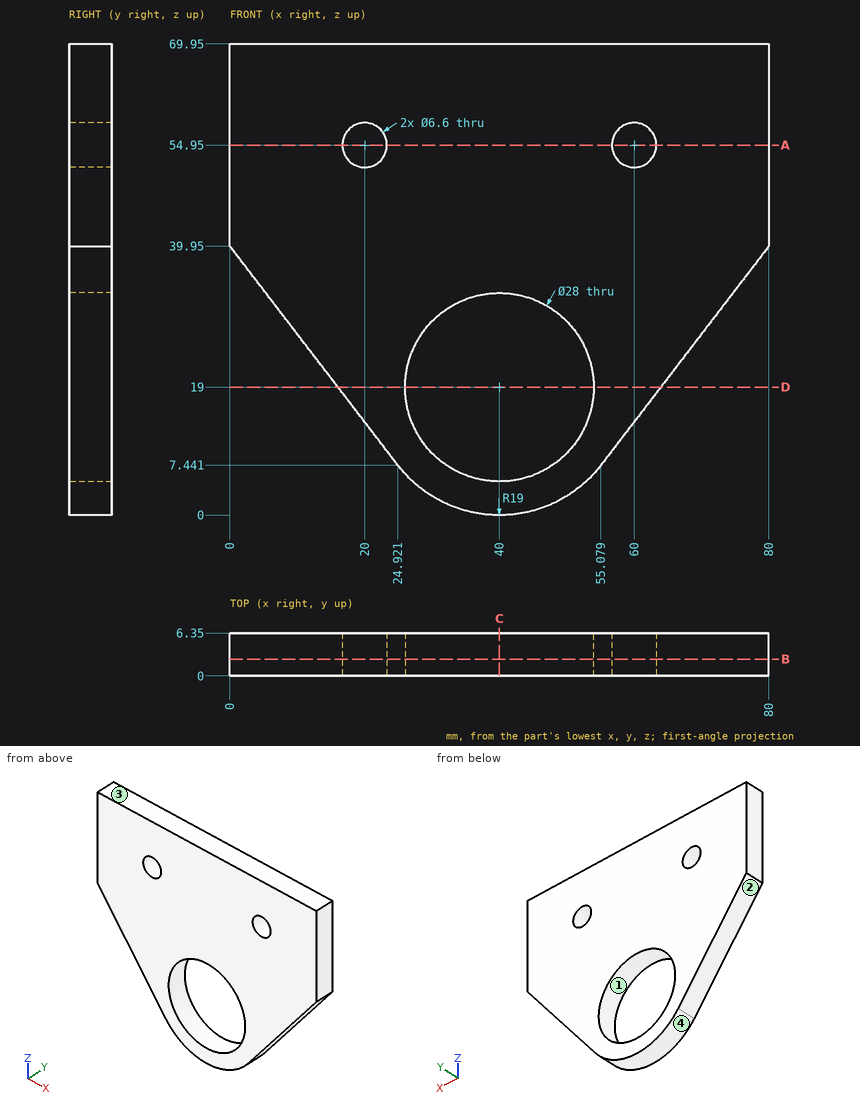
Can you work these out from the drawing? Everything is in mm from the part's minimum corner. Round coordinates to 2 decimals unless told otherwise and drop trailing zeros. Order: outer loops, then holes, each group sorted by start corner. A loop starts at its lowest first (then second) coordinate and runs counter-clockwise, first axis right, second up. Notation, with made-up numbers: M 9.25,42 L 32.25,42 A15 cw 32.25,63 Z; hole C -16,58 d5. An arc over 180 degrees is marked long. Answer as CSV lines item,"result".
Item 1: Imagine slicing it at A-A on z = 54.95. List the corners of the cut face in (x, y) for me, and give its area (3 significant figures).
From the geometry:
outline,"M 0,0 L 16.7,0 L 16.7,6.35 L 0,6.35 Z; M 23.3,0 L 56.7,0 L 56.7,6.35 L 23.3,6.35 Z; M 63.3,0 L 80,0 L 80,6.35 L 63.3,6.35 Z"
area,"424 mm2"
Item 2: Imagine slicing it at C-C on x = 40. List the corners of the cut face in (y, z) for me.
From the geometry:
outline,"M 0,0 L 6.35,0 L 6.35,5 L 0,5 Z; M 0,33 L 6.35,33 L 6.35,69.95 L 0,69.95 Z"
Item 3: We'd pull the mould along X, two halves only. Please class the marked faces 1, 2, 3 and 4: +X half, -X half, draft (parallel to the pull), parting line (faces both ways), or undercut.
From the geometry:
face 1,"undercut"
face 2,"-X half"
face 3,"draft"
face 4,"parting line"
Item 4: For pin 1 (1.5 mm diameter, centred on x = 68, y = 4, fed in from -Z), with a flat end and sliding along its axis, tell me the tip position at first contact or that it passes through.
From the geometry:
pin 1,"z = 23.32"
Item 5: Please list where these lines run through material, in increasing order: L1, parallel to X at y = 2.75, z = 54.95; L2, parallel to Z at x = 40, y = 4; L3, parallel to X at y = 0.75, z = 18 (1 decimal). Write a range as [from, to].
From the geometry:
L1,"[0, 16.7], [23.3, 56.7], [63.3, 80]"
L2,"[0, 5], [33, 69.95]"
L3,"[16.8, 26], [54, 63.2]"
Item 6: Imagine slicing it at D-D on z = 19. List the corners of the cut face in (x, y) for me.
From the geometry:
outline,"M 16.06,0 L 26,0 L 26,6.35 L 16.06,6.35 Z; M 54,0 L 63.94,0 L 63.94,6.35 L 54,6.35 Z"
Item 7: Imagine slicing it at B-B on y = 2.5. List the corners of the cut face in (x, z) for me.
From the geometry:
outline,"M 0,39.95 L 24.92,7.44 A19 ccw 55.08,7.44 L 80,39.95 L 80,69.95 L 0,69.95 Z; hole C 20,54.95 d6.6; hole C 40,19 d28; hole C 60,54.95 d6.6"
